Verification items for the finished model (mm, model axes). Face numbers are marked on the shaded views. A direction names the side the tool comes from. Round coordinates to 2 decimals unless told otherwise and drop trailing zeros. Write item = value, one per line. Start each with the question number.
Autodesk Inventor part; units mm, degrees
ref_plane "Top Plane" through (-7.3, 8.6, -7.3) normal (0, 1, 0) x (1, 0, 0)
ref_plane "YZ Plane" through (0, 0, 0) normal (1, 0, 0) x (0, 1, 0)
ref_plane "XZ Plane" through (0, 0, 0) normal (0, 1, 0) x (-1, 0, 0)
sketch "Base Loop" plane through (0, 0, 0) normal (0, 1, 0) x (-1, 0, 0)
  line L0 (-7.3, 7.3) -> (7.3, 7.3)
  line L1 (7.3, 7.3) -> (7.3, -7.3)
  line L2 (7.3, -7.3) -> (-7.3, -7.3)
  line L3 (-7.3, -7.3) -> (-7.3, 7.3)
  line L4 (-7.3, 7.3) -> (7.3, -7.3) construction
  line L5 (7.3, 7.3) -> (-7.3, -7.3) construction
  point P0 (0, 0)
  point P1 (0, 0)
  point P2 (0, 0)
  dimension "d0" = 14.6
  dimension "d1" = 14.6
ref_plane "Mid Plane" through (-7.3, 2, -7.3) normal (0, 1, 0) x (1, 0, 0)
ref_plane "Base Plane" through (-7.3, 0, -7.3) normal (0, 1, 0) x (1, 0, 0)
sketch "Mid Loop" plane through (-7.3, 2, -7.3) normal (0, 1, 0) x (1, 0, 0)
  line L0 (15.1, -15.1) -> (-0.5, -15.1)
  line L1 (-0.5, -15.1) -> (-0.5, 0.5)
  line L2 (-0.5, 0.5) -> (15.1, 0.5)
  line L3 (15.1, 0.5) -> (15.1, -15.1)
  line L4 (15.1, -15.1) -> (-0.5, 0.5) construction
  line L5 (-0.5, -15.1) -> (15.1, 0.5) construction
  point P0 (7.3, -7.3)
  dimension "d3" = 15.6
  dimension "d4" = 15.6
ref_plane "Top Plane" through (-7.3, 8.6, -7.3) normal (0, 1, 0) x (1, 0, 0)
sketch "Top Loop" plane through (-7.3, 8.6, -7.3) normal (0, 1, 0) x (1, 0, 0)
  line L0 (13.3, -13.3) -> (1.3, -13.3)
  line L1 (1.3, -13.3) -> (1.3, -1.3)
  line L2 (1.3, -1.3) -> (13.3, -1.3)
  line L3 (13.3, -1.3) -> (13.3, -13.3)
  line L4 (13.3, -13.3) -> (1.3, -1.3) construction
  line L5 (1.3, -13.3) -> (13.3, -1.3) construction
  point P0 (7.3, -7.3)
  dimension "d6" = 12
  dimension "d7" = 12
loft "Keyswitch Body" add profiles "Base Loop", "Mid Loop", "Top Loop"
sketch "Cut in profile" plane through (-6, 8.6, 6) normal (0, 1, 0) x (1, 0, 0)
  line L0 (8.75, 2.5) -> (3.25, 2.5)
  line L1 (3.25, 2.5) -> (3.25, 9.5)
  line L2 (3.25, 9.5) -> (8.75, 9.5)
  line L3 (8.75, 9.5) -> (8.75, 2.5)
  line L4 (8.75, 2.5) -> (3.25, 9.5) construction
  line L5 (3.25, 2.5) -> (8.75, 9.5) construction
  point P0 (6, 6)
  dimension "d17" = 7
  dimension "d18" = 5.5
extrude "Pole Cut in" cut sketch "Cut in profile" against normal blind 6.6
equation "\"d1\" = d0"
equation "\"d3\" = s_bwidth"
equation "\"d4\" = d3"
equation "\"d17\" = s_polebl"
equation "\"d18\" = s_polebw"
equation "\"k_width\" = 18.1"
equation "\"k_height\" = 18"
equation "\"k_taper1\" = 1.5"
equation "\"k_taper2\" = 0.5"
equation "\"k_radius\" = 6"
equation "\"k_wthick\" = 1.5"
equation "\"k_ribthick\" = 1.5"
equation "\"k_ribheight\" = 5"
equation "\"k_poleoff\" = 2.2625"
equation "\"k_poledia\" = 5.54"
equation "\"k_cmxw\" = 1.35"
equation "\"k_cmxl\" = 4.4"
equation "\"s_bwidth\" = 15.6"
equation "\"s_poleh\" = 3.6"
equation "\"s_polebw\" = 5.5"
equation "\"s_polebl\" = 7"
equation "\"b_rshift\" = 49.775"
equation "\"b_ctrl\" = 22.625"
equation "\"b_space\" = 117.65"
equation "\"b_height\" = 77.4"
equation "\"b_width\" = 286.5"
equation "\"b_lshift\" = 40.725"
equation "\"b_tab\" = 27.15"
equation "\"b_pad\" = 1"
equation "\"b_caps\" = 31.675"
equation "\"k_staper\" = 1"
equation "\"k_ltaper\" = 1.5"
equation "\"k_lradius\" = 6"
equation "\"k_sradius\" = 4"
equation "\"k_height_t\" = 16"
properties part number "keyswitch-base_cherrymx"
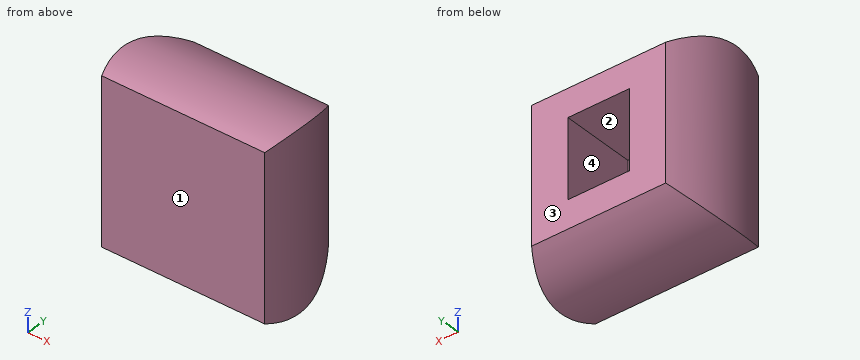
1) Scan lines: probe 1 along X at (y, z) = (7.75, 3.25); probe 2 along Y at (x, z) = (-2.5, -2.75); probe 3 along Z at (x, y) = (0, 6.5). Record each from-to range of solid material in increasing order.
2) Access from +Z, -Z, +X, -X, +Y, -Y to the whole of each face (thin tool, end or side, straight path). Record for the marked faces 3 and 4.
3) Release check for a two-part mould opening along Z. For the marked faces 1 and 2 record: pulls with the +Z half, pulls with the -Z half, needs draft (parallel to the pull), parting line crosses it, or undercut.
4) Gauge pin test, flat ends, axial feed: P1, Ø2, axis at y = 6, z = 0.5, coming from the -X side; P2, Ø5, axis at y = 2.5, z = -6, coming from the -X side; P3, Ø1.5, axis at x = 3, y = 6.5, coming from the -Z side; P4, Ø3, axis at x = 0.5, z = 0.5, coming from the +Y side. Record the tip position at first contact, or that the pin passes through.
Geometry results:
q1.probe_1 = -6.53 to -2.75, 2.75 to 6.53
q1.probe_2 = 0 to 2
q1.probe_3 = -7.16 to -3.5, 3.5 to 7.16
q2.face_3 = +Z, -Z, +X, -X, +Y
q2.face_4 = +Y
q3.face_1 = needs draft
q3.face_2 = undercut
q4.P1 = -7.65
q4.P2 = -7.87
q4.P3 = -7.44
q4.P4 = 2
